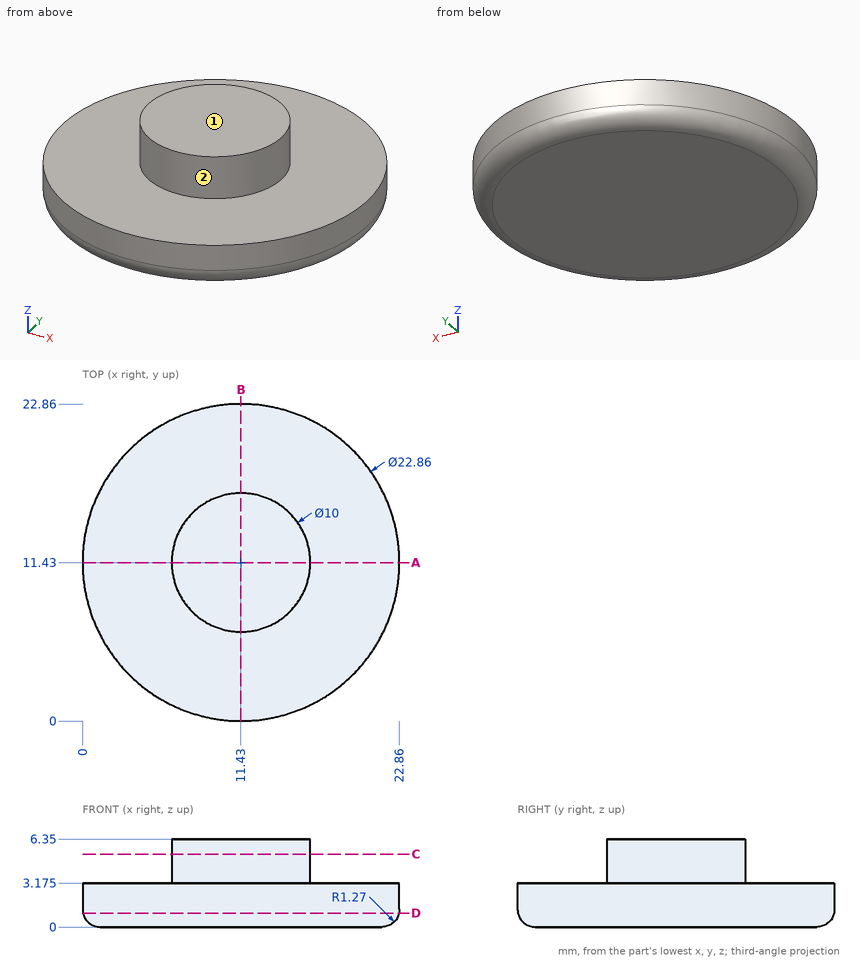
Design review of the part shown in the three views and the two pictorial views. Dimensions are in mm from the part's minimum x, y and z. A direction names the side the tool comes from. Round coordinates to 2 decimals unless told otherwise and drop trailing zeros. Write each loop counter-clockwise with the first axis right and the second up, starting at its lowest first coordinate (ties: lowest second). Pieces come first, ordered by that corner, then holes. Notation, with made-up numbers: (-7.5, -23) - (46.5, -23) arc R10 cw to (46.5, -18) - close; hole circle Ø4 at (-19.5, -24). An arc over 180 degrees is marked (long way). Answer as CSV lines item,"result". Start each with the question number.
(1) For line 1 (Z direction, x = 12, y = 17) (3 decimals); line 2 (X direction, y = 11.25, z = 5); line 3 (X direction, y = 11.25, z = 1.5), list the stretches that pass through material, from the lowest coordinate up.
(2) Add section D-D, the plane z = 1. State the section outline as (x, y) points.
(3) Add section A-A, the plane y = 11.43. State the section outline as (x, z) points (3 decimals), plus the area to 3 significant figures.
(4) Machinability: for the marked faces 1 and 2, which of the approach directions +Z, -Z, +X, -X, +Y, -Y give a long, thin tool a straight path to every point of the face, cutting with its end or side? Answer none if there is none.
(5) Add section C-C, the plane z = 5.25. State the section outline as (x, y) points, plus the area to 3 significant figures.
(6) For pin 1 (10 mm diameter, centred on x = 16.5, y = 8.5, fed in from +Z); pin 2 (1 mm diameter, centred on x = 18, y = 2.5, fed in from -Z); pin 3 (1 mm diameter, centred on x = 20.5, z = 2, fed in from -Y); pin 4 (2 mm diameter, centred on y = 4.5, z = 0.5, fed in from -X), all flat-tipped, find the tip position at first contact; note any pin that passes through.
From the geometry:
1,line 1,"z = 0 to 3.175"
1,line 2,"x = 6.43 to 16.43"
1,line 3,"x = 0 to 22.86"
2,outline,"circle Ø22.8 at (11.43, 11.43)"
3,outline,"(0, 1.27) arc R1.27 ccw to (1.27, 0) - (21.59, 0) arc R1.27 ccw to (22.86, 1.27) - (22.86, 3.175) - (16.43, 3.175) - (16.43, 6.35) - (6.43, 6.35) - (6.43, 3.175) - (0, 3.175) - close"
3,area,"104 mm²"
4,face 1,"+Z, +X, -X, +Y, -Y"
4,face 2,"+Z"
5,outline,"circle Ø10 at (11.43, 11.43)"
5,area,"78.5 mm²"
6,pin 1,"stops at z = 6.35"
6,pin 2,"stops at z = 0.07"
6,pin 3,"stops at y = 3.87"
6,pin 4,"stops at x = 1.77"
